Verification items for this drawing (mm, ordinates from the low corner). Round coordinates to 2 decimals unless told otherwise and drop trailing zeros. Order: outer loops, then holes, each group sorted by start corner. A loop starts at its lowest first (then second) coordinate and runs counter-clockwise, first axis right, second up. Notation, with made-up numbers: (0, 77.25) - (19, 77.25) arc R33 cw to (19, 115.25) - close; hole circle Ø1 at (59, 70). An arc over 180 degrees is marked (long way). Answer as CSV lines item,"result". Start each with the question number.
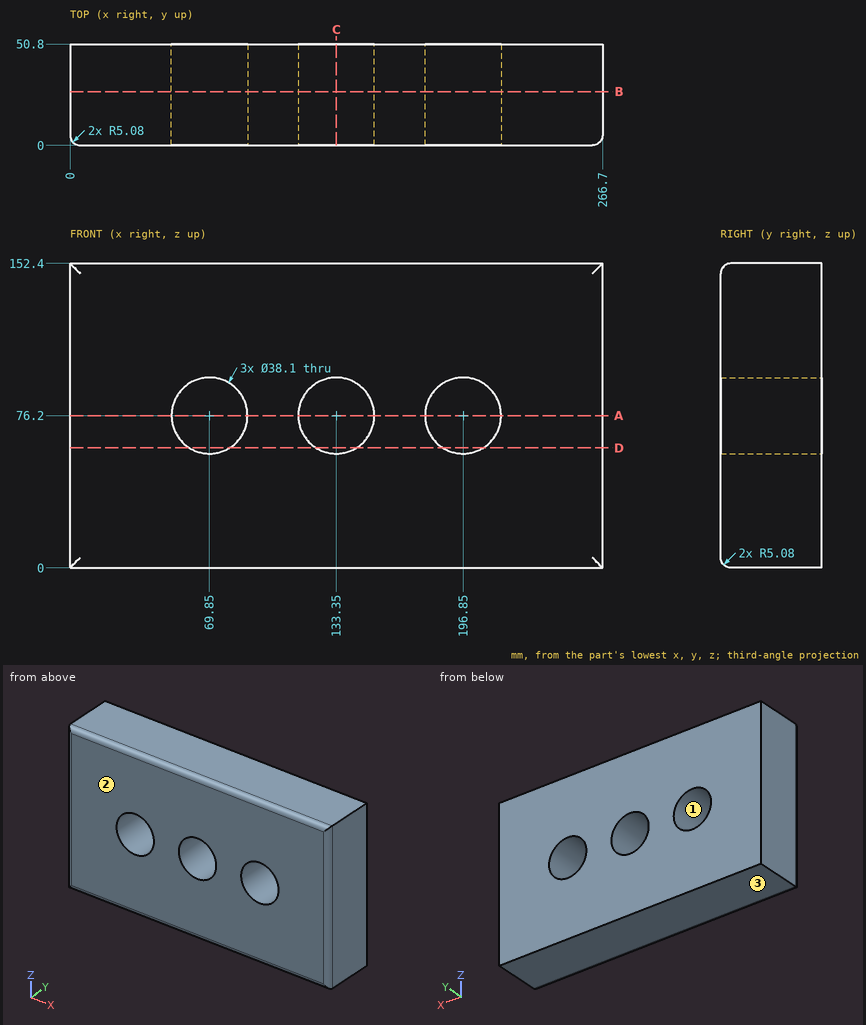
1. Section check A-A on z = 76.2. Record the boundary of the cut face in (x, y).
2. Section check B-B on y = 27. Record the boundary of the cut face in (x, z).
3. Section check D-D on z = 60. Record the boundary of the cut face in (x, y), plus the area to 3 significant figures.
4. Draft check along Z on the marked faces 1, 2 and 3. Enter one of: released by +Z, released by -Z, zero draft, split by the parting line, or undercut.
5. Section check C-C on x = 133.35. Record the boundary of the cut face in (y, z), plus the area to 3 significant figures.
6. Thickness scan on probe 1 along Z at (x, y) = (133, 13.5); probe 2 along X at (y, z) = (47, 89.5); probe 3 along X at (y, z) = (17, 72.5). Record the ranges inside material, lowest first.
Numbers:
1,outline,"(0, 5.08) arc R5.08 ccw to (5.08, 0) - (50.8, 0) - (50.8, 50.8) - (0, 50.8) - close; (88.9, 0) - (114.3, 0) - (114.3, 50.8) - (88.9, 50.8) - close; (152.4, 0) - (177.8, 0) - (177.8, 50.8) - (152.4, 50.8) - close; (215.9, 0) - (261.62, 0) arc R5.08 ccw to (266.7, 5.08) - (266.7, 50.8) - (215.9, 50.8) - close"
2,outline,"(0, 0) - (266.7, 0) - (266.7, 152.4) - (0, 152.4) - close; hole circle Ø38.1 at (69.85, 76.2); hole circle Ø38.1 at (133.35, 76.2); hole circle Ø38.1 at (196.85, 76.2)"
3,outline,"(0, 5.08) arc R5.08 ccw to (5.08, 0) - (59.83, 0) - (59.83, 50.8) - (0, 50.8) - close; (79.87, 0) - (123.33, 0) - (123.33, 50.8) - (79.87, 50.8) - close; (143.37, 0) - (186.83, 0) - (186.83, 50.8) - (143.37, 50.8) - close; (206.87, 0) - (261.62, 0) arc R5.08 ccw to (266.7, 5.08) - (266.7, 50.8) - (206.87, 50.8) - close"
3,area,"10,500 mm2"
4,face 1,"undercut"
4,face 2,"zero draft"
4,face 3,"released by -Z"
5,outline,"(0, 5.08) arc R5.08 ccw to (5.08, 0) - (50.8, 0) - (50.8, 57.15) - (0, 57.15) - close; (0, 95.25) - (50.8, 95.25) - (50.8, 152.4) - (5.08, 152.4) arc R5.08 ccw to (0, 147.32) - close"
5,area,"5,800 mm2"
6,probe 1,"z = 0 to 57.15, 95.25 to 152.4"
6,probe 2,"x = 0 to 56.21, 83.49 to 119.71, 146.99 to 183.21, 210.49 to 266.7"
6,probe 3,"x = 0 to 51.16, 88.54 to 114.66, 152.04 to 178.16, 215.54 to 266.7"
